Autodesk Inventor part; units mm, degrees
ref_plane "YZ Plane" through (0, 0, 0) normal (1, 0, 0) x (0, 1, 0)
ref_plane "XZ Plane" through (0, 0, 0) normal (0, 1, 0) x (-1, 0, 0)
ref_plane "XY Plane" through (0, 0, 0) normal (0, 0, 1) x (1, 0, 0)
sketch "Sketch1" plane through (0, 0, 0) normal (0, 1, 0) x (-1, 0, 0)
  line L0 (95, -95) -> (-95, -95)
  line L1 (-95, -95) -> (-95, 95)
  line L2 (-95, 95) -> (95, 95)
  line L3 (95, 95) -> (95, -95)
  line L4 (95, -95) -> (-95, 95) construction
  line L5 (-95, -95) -> (95, 95) construction
  point P0 (0, 0)
  point P1 (0, 0)
  point P2 (0, 0)
  dimension "d25" = 190
extrude "Extrusion1" add sketch "Sketch1" along normal blind 2.3813
sketch "Sketch2" plane through (0, 2.3813, 0) normal (0, 1, 0) x (1, 0, 0)
  line L0 (-95, -95) -> (95, -95)
  point P0 (0, 0)
  point P1 (0, -85)
  dimension "d26" = 10
hole "Hole1" at (0, 2.3813, 85) direction (0, -1, 0) diameter 5.5 end through all
pattern_circular "Circular Pattern1" count 4 over 360 about axis through (0, -10, 0) along (0, 1, 0) of "Hole1"
sketch "Sketch3" plane through (0, 0, 0) normal (0, -1, 0) x (1, 0, 0)
  circle A0 centre (-85, 0) radius 2.75
  circle A1 centre (0, -85) radius 2.75
  circle A2 centre (85, 0) radius 2.75
  circle A3 centre (0, 85) radius 2.75
  line L0 (-95, -95) -> (95, -95)
  line L1 (95, -95) -> (95, 95)
  line L2 (95, 95) -> (-95, 95)
  line L3 (-95, 95) -> (-95, -95)
  line L4 (0, 106.066) -> (106.066, 0)
  line L5 (106.066, 0) -> (0, -106.066)
  line L6 (0, -106.066) -> (-106.066, 0)
  line L7 (-106.066, 0) -> (0, 106.066)
  line L8 (-106.066, 0) -> (106.066, 0) construction
  line L9 (0, -106.066) -> (0, 106.066) construction
  point P0 (0, 0)
  point P1 (0, 0)
  point P2 (0, 0)
  dimension "d27" = 150
  dimension "d28" = 150
extrude "Extrusion2" cut sketch "Sketch3" against normal through all contours L6 L3 L7 L2 L4 L1 L5 L0 | L0 L5 L6 | L6 L7 L3 | L1 L4 L5 | L7 L4 L2 keep common part
equation "\"d7\" = suppourtPanelThickness"
equation "\"d28\" = d27"
equation "\"panelChamfer\" = 75"
equation "\"suppourtPanelThickness\" = 2.38125"
properties part number "separatingPanels" material "Polycarbonate, Clear"
Geometry check sheet. Reference: the model listing, model coordinates, mm. Coordinates: 2 decimals unless noted, no trailing zeros. Order: outer loops, then holes, each group sorted by start corner. A loop starts at its lowest first (then second) coordinate and runs counter-clockwise, first axis right, second up. Notation, with made-up numbers: (62.25, -20.75) - (97.25, -20.75) arc R10 cw to (97.25, -2.75) - close; hole circle Ø3 at (-21, -12). An arc over 180 degrees is marked (long way). Answer in a Markdown table with one row per item. Add a question column.
1. Section check A-A (z = 0). Enter the section's corners in (x, y).
2. Draft check along Z on faces 1 (the face through (-0.121, 1.174, 82.253)), 2 (the face through (-52.445, 1.174, -53.621)), 3 (the face through (-53.621, 1.174, 52.445)). Enter one of: +Z half, -Z half, draft (parallel to the pull), parting line (faces both ways), or undercut.
3. Section check B-B (y = 0.45). Enter the section's corners in (x, z), plus the area to 3 significant figures.
4. Section check D-D (z = 85). Enter the section's corners in (x, y), plus the area to 3 significant figures.
5. Gauge pin test, flat end, axial feed: pin 1 Ø4.5 at (x, z) = (0, 85) entering from -Y. Record the tip position at first contact, or that the pin passes through.
6. Material ranges on L1, parallel to Z at x = -85, y = 0.9; L2, parallel to X at y = 1.1, z = -31, recorded low to high. Write a range as [from, to].
7. Section check C-C (x = 85). Enter the section's corners in (y, z).
Data:
| question | item | result |
|---|---|---|
| 1 | outline | (-95, 0) - (-87.75, 0) - (-87.75, 2.38) - (-95, 2.38) - close; (-82.25, 0) - (82.25, 0) - (82.25, 2.38) - (-82.25, 2.38) - close; (87.75, 0) - (95, 0) - (95, 2.38) - (87.75, 2.38) - close |
| 2 | face 1 | undercut |
| 2 | face 2 | -Z half |
| 2 | face 3 | +Z half |
| 3 | outline | (-95, -11.07) - (-11.07, -95) - (11.07, -95) - (95, -11.07) - (95, 11.07) - (11.07, 95) - (-11.07, 95) - (-95, 11.07) - close; hole circle Ø5.5 at (-85, 0); hole circle Ø5.5 at (0, -85); hole circle Ø5.5 at (0, 85); hole circle Ø5.5 at (85, 0) |
| 3 | area | 21,900 mm² |
| 4 | outline | (-21.07, 0) - (-2.75, 0) - (-2.75, 2.38) - (-21.07, 2.38) - close; (2.75, 0) - (21.07, 0) - (21.07, 2.38) - (2.75, 2.38) - close |
| 4 | area | 87.2 mm² |
| 5 | pin 1 | passes through |
| 6 | L1 | z = [-21.07, -2.75], [2.75, 21.07] |
| 6 | L2 | x = [-75.07, 75.07] |
| 7 | outline | (0, -21.07) - (2.38, -21.07) - (2.38, -2.75) - (0, -2.75) - close; (0, 2.75) - (2.38, 2.75) - (2.38, 21.07) - (0, 21.07) - close |
